```python
from build123d import *

# Parameters (mm, degrees)
SKETCH1_R           = 80
BOSS_EXTRUDE1_DEPTH = 18
SKETCH2_R           = 12.5
CUT_EXTRUDE1_DEPTH  = 115.560027933
SKETCH3_R           = 9.571617906
CUT_EXTRUDE2_DEPTH  = 14.673866
CIRPATTERN1_START   = 3.326134057
CIRPATTERN1_DEPTH   = 14.673865943


# Read off the part's stored shape, not the designer's step: CirPattern1
with BuildPart() as part:
    # Sketch1 → Boss-Extrude1 (new body)
    with BuildSketch(Plane(origin=(0, 0, 0), x_dir=(1, 0, 0), z_dir=(0, 1, 0))):
        with Locations(Location((0, 0, 0), (0, 0, 270))):
            Circle(SKETCH1_R)
    extrude(amount=BOSS_EXTRUDE1_DEPTH)

    # Sketch2 → Cut-Extrude1 (cut, through all)
    with BuildSketch(Plane(origin=(0, 0, 0), x_dir=(1, 0, 0), z_dir=(0, 1, 0))):
        with Locations(Location((0, 0, 0), (0, 0, 270))):
            Circle(SKETCH2_R)
    extrude(amount=CUT_EXTRUDE1_DEPTH, mode=Mode.SUBTRACT)

    # Sketch3 → Cut-Extrude2 (cut)
    with BuildSketch(Plane(origin=(0, 18, 0), x_dir=(1, 0, 0), z_dir=(0, 1, 0))):
        with Locations((-15.612808267, 0)):
            Circle(SKETCH3_R)
    extrude(amount=-CUT_EXTRUDE2_DEPTH, mode=Mode.SUBTRACT)

    # CirPattern1 outline → CirPattern1 (cut)
    with BuildSketch(Plane(origin=(0, 0, 0), x_dir=(1, 0, 0), z_dir=(0, 1, 0)).offset(CIRPATTERN1_START)):
        with BuildLine():
            ThreePointArc((-9.876311403, -7.662145461), (-11.096255907, -8.43899426), (-12.419321601, -9.023165312))
            ThreePointArc((-12.419321601, -9.023165312), (-7.782415681, -23.951812621), (4.743758735, -14.599788162))
            ThreePointArc((4.743758735, -14.599788162), (20.374628767, -14.803034291), (15.351125734, 0))
            ThreePointArc((15.351125734, 0), (20.374628767, 14.803034291), (4.743758735, 14.599788162))
            ThreePointArc((4.743758735, 14.599788162), (-7.782415681, 23.951812621), (-12.419321601, 9.023165312))
            ThreePointArc((-12.419321601, 9.023165312), (-11.096255907, 8.43899426), (-9.876311403, 7.662145461))
            ThreePointArc((-9.876311403, 7.662145461), (12.5, 0), (-9.876311403, -7.662145461))
        make_face()
    extrude(amount=CIRPATTERN1_DEPTH, mode=Mode.SUBTRACT)


solid = part.part
```
Model file for the job. Use its own axes, mm. A direction names the side the tool comes from. Coordinates: 2 decimals unless noted, no trailing zeros. Loops run counter-clockwise (first coordinate to the right, second up) from the corner with the lowest first, then second, coordinate; pieces in that order, holes last. Notation, with made-up numbers: (-9.5, 50) -> (11.5, 50) arc R26 cw to (11.5, 85) -> close; hole circle Ø5 at (-33, 31.5). An arc over 180 degrees is marked (long way). Answer as a JSON object with one key per item and string values.
Q1. Probe probe 1 along Y at (x, z) = (-1, -14); probe 2 along X at (y, z) = (1, -8); probe 3 along X at (y, z) = (1.5, -11). List the from-to ranges inside material, lowest first.
Report:
{"probe 1": "y = 0 to 3.33", "probe 2": "x = -79.6 to -9.6, 9.6 to 79.6", "probe 3": "x = -79.24 to -5.94, 5.94 to 79.24"}
Q2. Cut at C-C (y = 14.75). List the corners of the cut face in (x, z).
Report:
{"outline": "circle Ø160 at (0, 0); hole (-12.42, -9.02) arc R9.57 ccw (long way) to (4.74, -14.6) arc R9.57 ccw (long way) to (15.35, 0) arc R9.57 ccw (long way) to (4.74, 14.6) arc R9.57 ccw (long way) to (-12.42, 9.02) arc R9.57 ccw (long way) to start"}
Q3. Cut at D-D (x = 68.5). List the corners of the cut face in (y, z).
Report:
{"outline": "(0, -41.32) -> (18, -41.32) -> (18, 41.32) -> (0, 41.32) -> close"}
Q4. Flat gauge pins, fed straight in: P1, Ø1, axis at x = -58, y = 2, coming from the +Z side; P2, Ø6, axis at y = 7.5, z = 23.5, coming from the +X side; P3, Ø20, axis at x = 0, z = 0, coming from the -Y side; P4, Ø4, axis at y = 6.5, z = 43.5, coming from the -X side. Where does each tip first touch, or does it go through?
Report:
{"P1": "stops at z = 55.62", "P2": "stops at x = 77.33", "P3": "passes through", "P4": "stops at x = -68.39"}
Q5. Cut at A-A (x = 0). List the corners of the cut face in (y, z).
Report:
{"outline": "(0, -80) -> (18, -80) -> (18, -23.12) -> (3.33, -23.12) -> (3.33, -12.5) -> (0, -12.5) -> close; (0, 12.5) -> (3.33, 12.5) -> (3.33, 23.12) -> (18, 23.12) -> (18, 80) -> (0, 80) -> close"}
Q6. Pull direction Z, two halves, no side cores. Call faces 3 (the cylindrical face through (-25.18, 10.77, -0.26)), 4 (the flat face through (19, 18, -1)), 5 (the cylindrical face through (-78.1, 8.87, -17.34)): released by +Z, released by -Z, zero draft, split by the parting line, or undercut.
Report:
{"face 3": "undercut", "face 4": "zero draft", "face 5": "split by the parting line"}
Q7. 3-axis set-ups, long thin cutter, end or side, ignore diameter. For faces 1 (the cylindrical face through (3.755, 1.64, 11.923)), 2 (the cylindrical face through (20.522, 10.56, -14.594)): which of +Z, -Z, +X, -X, +Y, -Y reach the whole face in a straight line?
Report:
{"face 1": "+Y, -Y", "face 2": "+Y"}
Q8. Cut at B-B (z = 3). List the corners of the cut face in (x, y).
Report:
{"outline": "(-79.94, 0) -> (-12.13, 0) -> (-12.13, 3.33) -> (-24.7, 3.33) -> (-24.7, 18) -> (-79.94, 18) -> close; (12.13, 0) -> (79.94, 0) -> (79.94, 18) -> (19.94, 18) -> (19.94, 3.33) -> (12.13, 3.33) -> close"}
